Can you work these out from the drawing? Everything is in mm from the part's minimum corner. A direction names the side the tool comes from. Give positions to 0.01 mm unless a question says otherwise; leave off trailing zeros. Order: outer loops, then holes, each group sorted by start corner. A loop starts at its lowest first (then second) coordinate and runs counter-clockwise, first axis right, second up. Notation, with made-up numbers: (-0.75, 43.5) -> (36.25, 43.5) arc R21 cw to (36.25, 66.5) -> close; hole circle Ø10 at (2, 52). An arc over 180 degrees is marked (long way). One line per item, written item: value.
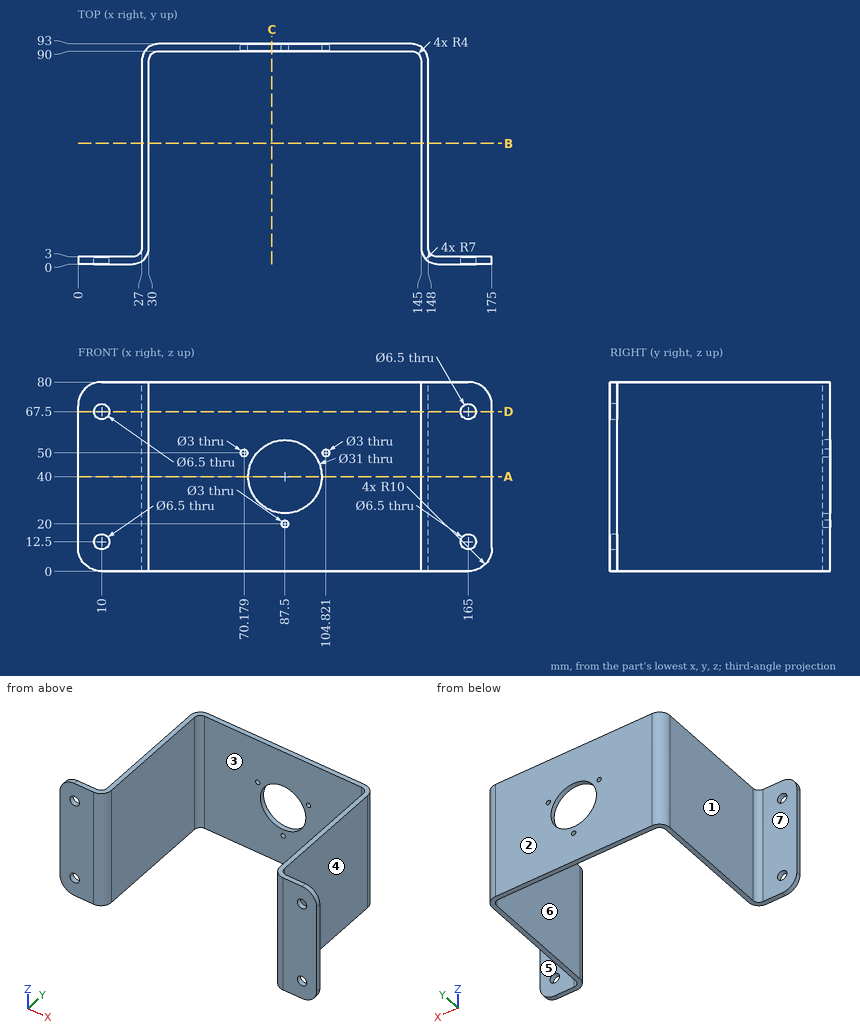
1) Suppose I cut it at B-B, the plane y = 51. Write out the boundary of the cut face in (x, z), then the cut area to 3 significant figures.
Answer below:
outline: (27, 0) -> (30, 0) -> (30, 80) -> (27, 80) -> close; (145, 0) -> (148, 0) -> (148, 80) -> (145, 80) -> close
area: 480 mm2
2) We'd pull the mould along X, two halves only. Please class the marked faces 1, 2, 3 and 4: +X half, -X half, draft (parallel to the pull), parting line (faces both ways), or undercut.
Answer below:
face 1: -X half
face 2: draft
face 3: undercut
face 4: +X half
3) Suppose I cut it at C-C, the plane x = 82. Write out the boundary of the cut face in (y, z).
Answer below:
outline: (90, 0) -> (93, 0) -> (93, 25.51) -> (90, 25.51) -> close; (90, 54.49) -> (93, 54.49) -> (93, 80) -> (90, 80) -> close
4) Suppose I cut it at D-D, the plane z = 67.5. Write out the boundary of the cut face in (x, y).
Answer below:
outline: (0, 0) -> (6.75, 0) -> (6.75, 3) -> (0, 3) -> close; (13.25, 0) -> (23, 0) arc R7 ccw to (30, 7) -> (30, 86) arc R4 cw to (34, 90) -> (141, 90) arc R4 cw to (145, 86) -> (145, 7) arc R7 ccw to (152, 0) -> (161.75, 0) -> (161.75, 3) -> (152, 3) arc R4 cw to (148, 7) -> (148, 86) arc R7 ccw to (141, 93) -> (34, 93) arc R7 ccw to (27, 86) -> (27, 7) arc R4 cw to (23, 3) -> (13.25, 3) -> close; (168.25, 0) -> (175, 0) -> (175, 3) -> (168.25, 3) -> close
5) For P1, Ø4, axis at x = 165, z = 67.5, coming from the -Y side; P2, Ø23.5, axis at y = 62, z = 27.5, coming from the -X side; P3, Ø7, axis at x = 7, z = 41.5, coming from the +Y side; P4, Ø3, axis at y = 83.5, z = 18, coming from the +X side, each with a flat end and sliding along its axis, tell me the tip position at first contact or that it passes through.
Answer below:
P1: passes through
P2: stops at x = 27
P3: stops at y = 3
P4: stops at x = 148
6) If I drill on line 1 along Z through (x, y) = (165, 0.8); line 2 along X through (y, z) = (81.5, 36); line 3 along X through (y, z) = (90.9, 50) (1 decimal), over which ranges is the centre line in solid material (lowest first)?
Answer below:
line 1: z = 0 to 9.25, 15.75 to 64.25, 70.75 to 80
line 2: x = 27 to 30, 145 to 148
line 3: x = 29 to 68.7, 71.7 to 75.7, 99.3 to 103.3, 106.3 to 146
7) Suppose I cut it at A-A, the plane z = 40. Write out the boundary of the cut face in (x, y).
Answer below:
outline: (0, 0) -> (23, 0) arc R7 ccw to (30, 7) -> (30, 86) arc R4 cw to (34, 90) -> (72, 90) -> (72, 93) -> (34, 93) arc R7 ccw to (27, 86) -> (27, 7) arc R4 cw to (23, 3) -> (0, 3) -> close; (103, 90) -> (141, 90) arc R4 cw to (145, 86) -> (145, 7) arc R7 ccw to (152, 0) -> (175, 0) -> (175, 3) -> (152, 3) arc R4 cw to (148, 7) -> (148, 86) arc R7 ccw to (141, 93) -> (103, 93) -> close
8) For the marked faces 5, 6 and 7, which set-ups out of +Z, -Z, +X, -X, +Y, -Y let a thin tool reach every point of the face, with its end or its side?
Answer below:
face 5: +Z, -Z, +X, +Y
face 6: +Z, -Z, -Y
face 7: +Z, -Z, -X, +Y
